CAD build for the part. Positions are in the model's coordinates, mm. A direction names the side the tool comes from. Coordinates: 2 decimals unless noted, no trailing zeros. Order: outer loops, then holes, each group sorted by start corner. A loop starts at its lowest first (then second) coordinate and runs counter-clockwise, first axis right, second up. Notation, with made-up numbers: (7.25, 46.5) - (22.25, 46.5) arc R21 cw to (22.25, 69.5) - close; hole circle Ø11 at (85.25, 75.25). An arc over 180 degrees is marked (long way). Use one line per item in the form item = value.
```python
from build123d import *

# Parameters (mm, degrees)
BOX006_W     = 190
BOX006_H     = 190
BOX006_DEPTH = 15
BOX005_W     = 200
BOX005_H     = 200
BOX005_DEPTH = 10


with BuildPart() as cube006:
    # Box006 → Box006 (new body)
    with BuildSketch(Plane(origin=(5, 5, 91), x_dir=(1, 0, 0), z_dir=(0, 0, 1))):
        with Locations((95, 95)):
            Rectangle(BOX006_W, BOX006_H)
    extrude(amount=BOX006_DEPTH)


with BuildPart() as lid:
    # Box005 → Box005 (new body)
    with BuildSketch(Plane.XY.offset(96)):
        with Locations((100, 100)):
            Rectangle(BOX005_W, BOX005_H)
    extrude(amount=BOX005_DEPTH)

    # Fusion002: union Cube006
    add(cube006.part)


solid = lid.part
```
Item 1: Drill centre line: line 1 (X direction, y = 124, z = 92.75). Where is it in solid material? Low to high. Write a range as [from, to].
Derived:
line_1 = [5, 195]
Item 2: Cut at C-C, the plane z = 93.5. Write the cut outline in (x, y), plus the area to 3 significant figures.
Derived:
outline = (5, 5) - (195, 5) - (195, 195) - (5, 195) - close
area = 36,100 mm²
Item 3: 3-axis set-ups, long thin cutter, end or side, ignore diameter. For faces 1 (the face through (195, 99, 93)), 2 (the face through (5, 99, 93)), 3 (the face through (99, 195, 93)), 4 (the face through (99, 5, 93)): which of +Z, -Z, +X, -X, +Y, -Y reach the whole face in a straight line?
Derived:
face_1 = -Z, +X, +Y, -Y
face_2 = -Z, -X, +Y, -Y
face_3 = -Z, +X, -X, +Y
face_4 = -Z, +X, -X, -Y
Item 4: Drop flat-ended pins along their axis: pin 1 (4 mm diameter, centred on y = 118.5, z = 92.5, fed in from +X); pin 2 (6 mm diameter, centred on y = 133.5, z = 96.5, fed in from -X); pin 3 (1.5 mm diameter, centred on y = 132.5, z = 93.5, fed in from -X); pin 4 (1.5 mm diameter, centred on x = 120, z = 93.5, fed in from +Y). Give the stop position or say it passes through.
Derived:
pin_1 = 195
pin_2 = 0
pin_3 = 5
pin_4 = 195
Item 5: Cut at A-A, the plane y = 96. Write the cut outline in (x, z).
Derived:
outline = (0, 96) - (5, 96) - (5, 91) - (195, 91) - (195, 96) - (200, 96) - (200, 106) - (0, 106) - close
